from build123d import *

# Parameters (mm, degrees)
SKETCH1_W           = 241.3
SKETCH1_H           = 38.1
BOSS_EXTRUDE1_DEPTH = 6.35
SKETCH2_R           = 3.81
CUT_EXTRUDE1_DEPTH  = 7.35
SKETCH3_W           = 241.3
SKETCH3_H           = 12.7
BOSS_EXTRUDE2_DEPTH = 139.7
CUT_EXTRUDE4_DEPTH  = 242.3
BOSS_EXTRUDE5_DEPTH = 241.3


with BuildPart() as part:
    # Sketch1 → Boss-Extrude1 (new body)
    with BuildSketch(Plane(origin=(0, 0, 0), x_dir=(1, 0, 0), z_dir=(0, 1, 0))):
        with Locations((24.806115108, 12.928417266)):
            Rectangle(SKETCH1_W, SKETCH1_H)
    extrude(amount=BOSS_EXTRUDE1_DEPTH)

    # Sketch2 → Cut-Extrude1 (cut, through all)
    with BuildSketch(Plane(origin=(0, 6.35, 0), x_dir=(1, 0, 0), z_dir=(0, 1, 0))):
        with Locations((-89.493884892, 12.928417266)):
            Circle(SKETCH2_R)
        with Locations((-64.093884892, 12.928417266)):
            Circle(SKETCH2_R)
        with Locations((113.706115108, 12.928417266)):
            Circle(SKETCH2_R)
        with Locations((139.106115108, 12.928417266)):
            Circle(SKETCH2_R)
    extrude(amount=-CUT_EXTRUDE1_DEPTH, mode=Mode.SUBTRACT)

    # Sketch3 → Boss-Extrude2 (add)
    with BuildSketch(Plane(origin=(0, 6.35, 0), x_dir=(1, 0, 0), z_dir=(0, 1, 0))):
        with Locations((24.806115108, 25.628417266)):
            Rectangle(SKETCH3_W, SKETCH3_H)
    extrude(amount=BOSS_EXTRUDE2_DEPTH)

    # Sketch8 → Cut-Extrude4 (cut, through all)
    with BuildSketch(Plane.ZY.offset(95.843884892)):
        Polygon((-19.278417266, 146.05), (-31.978417266, 146.05), (-31.978417266, 133.35), align=None)
        Polygon((-31.978417266, 133.35), (-31.978417266, 146.05), (-19.278417266, 146.05), (-19.278417266, 148.59), (-34.518417266, 148.59), (-34.518417266, 133.35), align=None)
    extrude(amount=-CUT_EXTRUDE4_DEPTH, mode=Mode.SUBTRACT)

    # Sketch9 → Boss-Extrude5 (add)
    with BuildSketch(Plane.ZY.offset(95.843884892)):
        Polygon((-30.054724611, 138.865795103), (-12.094212369, 156.826307345), (-10.298161145, 155.030256121), (-28.258673387, 137.069743879), align=None)
    extrude(amount=-BOSS_EXTRUDE5_DEPTH)


solid = part.part
Geometry check sheet. Reference: the model listing, model coordinates, mm. A direction names the side the tool comes from. Give positions to 0.01 mm unless a question says otherwise; leave off trailing zeros. Loops run counter-clockwise (first coordinate to the right, second up) from the corner with the lowest first, then second, coordinate; pieces in that order, holes last. Notation, with made-up numbers: M -35.75,89.25 L 21.25,89.25 A35 ccw 21.25,121.25 Z; hole C 77.25,-3 d10. An arc over 180 degrees is marked long. Write each question's results on one line, items separated by ' | '.
1) Section check B-B, the plane y = 27.5. Record the boundary of the cut face in (x, z), plus the area to 3 significant figures.
Answers follow:
outline: M -95.84,-31.98 L 145.46,-31.98 L 145.46,-19.28 L -95.84,-19.28 Z | area: 3,060 mm2
2) Tool access check on faces 4 (the face through (23, 3, 6.122)), 5 (the face through (-66.902, 3.219, -15.503)), 6 (the face through (23.12, 150.6, -14.73)). Record the directions out of +Z, -Z, +X, -X, +Y, -Y that give a thin tool (end or side, any length) a straight path to the whole face; none if there is none.
Answers follow:
face 4: +Z, +X, -X, +Y, -Y | face 5: -Y | face 6: +Z, +X, -X
3) Gauge pin test, flat ends, axial feed: pin 1 (2 mm diameter, centred on x = 39.5, z = -5.5, fed in from +Y); pin 2 (2 mm diameter, centred on x = -39, y = 76, fed in from +Z); pin 3 (4.5 mm diameter, centred on x = -89.49, z = -12.93, fed in from -Y). Record the tip position at first contact, or that the pin passes through.
Answers follow:
pin 1: y = 6.35 | pin 2: z = -19.28 | pin 3: y = 150.15
4) Section check C-C, the plane z = 2. Record the boundary of the cut face in (x, y), plus the area to 3 significant figures.
Answers follow:
outline: M -95.84,0 L 145.46,0 L 145.46,6.35 L -95.84,6.35 Z | area: 1,530 mm2
5) Thickness scan on line 1 (Y direction, x = -2, z = -5); line 2 (Z direction, x = -17, y = 77); line 3 (Y direction, x = 31, z = -26). Record the ranges inside material, lowest first.
Answers follow:
line 1: 0 to 6.35 | line 2: -31.98 to -19.28 | line 3: 0 to 142.92
6) Release check for a two-part mould opening along Z. For faces 1 (the face through (23, 66, -31.978)), 2 (the face through (-95.844, 67, -26)), 3 (the face through (117.34, 3.22, -14.07)) record: +Z half, -Z half, draft (parallel to the pull), parting line (faces both ways), or undercut.
Answers follow:
face 1: -Z half | face 2: draft | face 3: undercut
7) Section check A-A, the plane x = -44.5. Record the boundary of the cut face in (y, z), plus the area to 3 significant figures.
Answers follow:
outline: M 0,-31.98 L 133.35,-31.98 L 137.07,-28.26 L 138.87,-30.05 L 156.83,-12.09 L 155.03,-10.3 L 146.05,-19.28 L 6.35,-19.28 L 6.35,6.12 L 0,6.12 Z | area: 2,000 mm2
